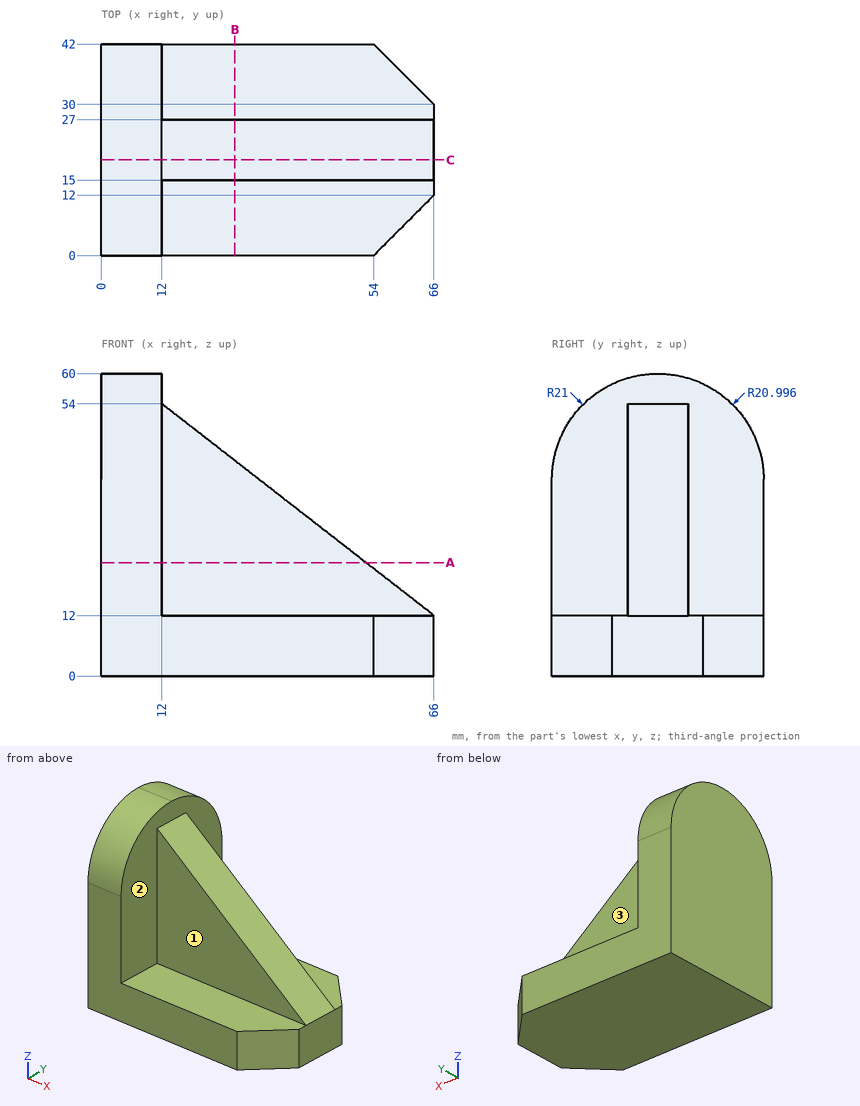
Drawing for the job (mm, zero at the part's lowest x, y, z). A direction names the side the tool comes from. Give positions to 0.01 mm unless a question says otherwise; leave off trailing zeros. Order: outer loops, then holes, each group sorted by start corner. A loop starts at its lowest first (then second) coordinate and runs counter-clockwise, first axis right, second up. Notation, with made-up numbers: (14, 61) - (37, 61) arc R29 cw to (37, 96) - close; hole circle Ø6 at (61.5, -35.75). An arc over 180 degrees is marked (long way). Use one line per item in the form item = value.
Item 1: Pin check, flat tips, straight feed: pin 1 Ø5 at (y, z) = (17, 10.5) entering from -X; pin 2 Ø6 at (x, z) = (34, 34) entering from +Y; pin 3 Ø3 at (x, z) = (58, 15.5) entering from -Y; pin 4 Ø7.5 at (x, y) = (42.5, 4) entering from +Z. Stop position of each tip, or through.
Solution:
pin_1 = 0
pin_2 = 27
pin_3 = 15
pin_4 = 12
Item 2: Slice it at B-B on x = 26.5. Give the cut face in (y, z).
Solution:
outline = (0, 0) - (42, 0) - (42, 12) - (27, 12) - (27, 42.72) - (15, 42.72) - (15, 12) - (0, 12) - close
Item 3: Probe probe 1 along Y at (x, z) = (47, 18.5); probe 2 along X at (y, z) = (9, 44). List the from-to ranges inside material, lowest first. Write a range as from..to.
Solution:
probe_1 = 15..27
probe_2 = 0..12
Item 4: Which spindle directions (+Z, -Z, +X, -X, +Y, -Y) get a long thin tool onto all of the face, cutting with end or side? Do the marked faces 1, 2 and 3. Say none if no direction does.
Solution:
face_1 = +Z, +X, -Y
face_2 = +Z, +X
face_3 = +Z, +X, +Y
Item 5: Slice it at C-C on y = 19. Give the cut face in (x, z), and give its area (3 significant figures).
Solution:
outline = (0, 0) - (66, 0) - (66, 12) - (12, 54) - (12, 59.9) - (0, 59.9) - close
area = 2,500 mm2
Item 6: Slice it at A-A on z = 22.5. Give the cut face in (x, y).
Solution:
outline = (0, 0) - (12, 0) - (12, 15) - (52.5, 15) - (52.5, 27) - (12, 27) - (12, 42) - (0, 42) - close
